Build history of the part. All positions in model axes, mm. A direction names the side the tool comes from. Give positions to 0.01 mm unless a question says otherwise; leave off trailing zeros. Write each loop counter-clockwise with the first axis right and the second up, starting at its lowest first coordinate (ties: lowest second). Pieces come first, ordered by that corner, then holes. Notation, with made-up numbers: (8.25, 70.25) - (42.25, 70.25) arc R29 cw to (42.25, 98.25) - close; hole circle Ø5 at (-30, 32.25). An arc over 180 degrees is marked (long way). Use one line per item in the form item = value. Start each with the question number.
from build123d import *

# Parameters (mm, degrees)
SKICA2_W                 = 63.5
SKICA2_H                 = 53.6
P_IDAT_VYSUNUT_M1_DEPTH  = 5
SKICA3_W                 = 63.5
SKICA3_H                 = 13
P_IDAT_VYSUNUT_M2_DEPTH  = 7.4
SKICA5_R                 = 8.5
ODEBRAT_VYSUNUT_M1_DEPTH = 74
ZKOSEN_1_SIZE            = 3
ZKOSEN_1_SIZE_2          = 3.575260778
ZAOBLIT1_R               = 2


with BuildPart() as part:
    # Skica2 → Přidat vysunutím1 (new body)
    with BuildSketch(Plane.XY):
        with Locations((6.211756064, 35.331333862)):
            Rectangle(SKICA2_W, SKICA2_H)
    extrude(amount=P_IDAT_VYSUNUT_M1_DEPTH)

    # Skica3 → Přidat vysunutím2 (add)
    with BuildSketch(Plane.XY.offset(5)):
        with Locations((6.211756064, 15.031333862)):
            Rectangle(SKICA3_W, SKICA3_H)
    extrude(amount=P_IDAT_VYSUNUT_M2_DEPTH)

    # Skica5 → Odebrat vysunutím1 (cut)
    with BuildSketch(Plane(origin=(0, 0, 0), x_dir=(-1, 0, 0), z_dir=(0, 0, -1))):
        with Locations((-17.961756064, 30.531333862)):
            Circle(SKICA5_R)
        with Locations((8.538243936, 30.531333862)):
            Circle(SKICA5_R)
    extrude(amount=-ODEBRAT_VYSUNUT_M1_DEPTH, mode=Mode.SUBTRACT)

    # Zkosení1
    # the kernel refuses this chamfer: 3.575260778, 3 mm, written as the material it takes off along each edge
    with BuildSketch(Plane(origin=(17.961756064, 30.531333862, 5), x_dir=(-1, 0, 0), z_dir=(0, -1, 0))) as zkosen_1_piece_1_section:
        Polygon((8.5 + ZKOSEN_1_SIZE, 0), (8.5, ZKOSEN_1_SIZE_2), (8.5, 0), align=None)
    zkosen_1_piece_1 = revolve(axis=Axis((17.961756064, 30.531333862, 5), (0, 0, -1)), mode=Mode.PRIVATE)
    zkosen_1_piece_1 = split(zkosen_1_piece_1, bisect_by=Plane(origin=(27.909166998, 21.531333862, 3.256497077), z_dir=(0, 1, 0)), keep=Keep.TOP, mode=Mode.PRIVATE)
    add(zkosen_1_piece_1, mode=Mode.SUBTRACT)
    with BuildSketch(Plane(origin=(-8.538243936, 30.531333862, 5), x_dir=(-1, 0, 0), z_dir=(0, -1, 0))) as zkosen_1_piece_2_section:
        Polygon((8.5 + ZKOSEN_1_SIZE, 0), (8.5, ZKOSEN_1_SIZE_2), (8.5, 0), align=None)
    zkosen_1_piece_2 = revolve(axis=Axis((-8.538243936, 30.531333862, 5), (0, 0, -1)), mode=Mode.PRIVATE)
    zkosen_1_piece_2 = split(zkosen_1_piece_2, bisect_by=Plane(origin=(1.409166998, 21.531333862, 3.256497077), z_dir=(0, 1, 0)), keep=Keep.TOP, mode=Mode.PRIVATE)
    add(zkosen_1_piece_2, mode=Mode.SUBTRACT)

    # Zaoblit1
    # the kernel refuses this fillet: 2 mm, written as the material it takes off along each edge
    with BuildSketch(Plane(origin=(17.961756064, 30.531333862, 0), x_dir=(-1, 0, 0), z_dir=(0, -1, 0))) as zaoblit1_piece_1:
        with BuildLine():
            CenterArc((10.415482978, -2), ZAOBLIT1_R, 90, 73.283856072)
            Line((8.5, -1.424739222), (8.46169034, -1.413234006))
            ThreePointArc((8.46169034, -1.413234006), (8.46, -0.712369611), (8.46, 0))
            Line((8.46, 0), (8.5, 0.04))
            Line((8.5, 0.04), (10.415482978, 0.04))
            Line((10.415482978, 0.04), (10.415482978, 0))
        make_face()
    revolve(axis=Axis((17.961756064, 30.531333862, 0), (0, 0, -1)), mode=Mode.SUBTRACT)
    with BuildSketch(Plane(origin=(-8.538243936, 30.531333862, 0), x_dir=(-1, 0, 0), z_dir=(0, -1, 0))) as zaoblit1_piece_2:
        with BuildLine():
            CenterArc((10.415482978, -2), ZAOBLIT1_R, 90, 73.283856072)
            Line((8.5, -1.424739222), (8.46169034, -1.413234006))
            ThreePointArc((8.46169034, -1.413234006), (8.46, -0.712369611), (8.46, 0))
            Line((8.46, 0), (8.5, 0.04))
            Line((8.5, 0.04), (10.415482978, 0.04))
            Line((10.415482978, 0.04), (10.415482978, 0))
        make_face()
    revolve(axis=Axis((-8.538243936, 30.531333862, 0), (0, 0, -1)), mode=Mode.SUBTRACT)


solid = part.part
(1) Cut at C-C, the plane y = 26. State how many separate pieces and enclosed holes the cut face has, then the cut area to 3 significant figures.
(2) Wall check: line 1 (X direction, y = 26, z = 2.5); line 2 (Z direction, x = 3, y = 44.5); line 3 (X direction, y = 36, z = 0.5). Give the ranges that are in metal, low to high. Write a range as from..to.
(3) Cut at A-A, the plane x = 5.5. Give the cut face in (y, z), then the cut area to 3 significant figures.
(4) Pin check, flat tips, straight feed: pin 1 Ø5 at (y, z) = (52, 9) entering from +X; pin 2 Ø4 at (x, z) = (-3.5, 8.5) entering from +Y. Stop position of each tip, or through.
(5) Cut at B-B, the plane z = 4.25. Give the cut face in (x, y), then the cut area to 3 significant figures.
(6) Cut at D-D, the plane z = 7.5. Give the cut face in (x, y), then the cut area to 4 significant figures.
(7) Which spindle directions (+Z, -Z, +X, -X, +Y, -Y) get a long thin tool onto all of the face, cutting with end or side? Do faces 1 (the flat face through (6, 47, 5)), 2 (the flat face through (6, 36, 0)), 3 (the flat face through (6, 21.531, 8)). Say none if no direction does.
(8) Two-plate mould, pull along Y, no slides. Class faces 4 (the conical face through (19.087, 39.103, 1.598)), 5 (the flat face through (6, 62.131, 2)), 6 (the flat face through (37.962, 29, 3)): +Y half, -Y half, draft (parallel to the pull), parting line (faces both ways), or undercut.
Solution:
q1.separate_pieces = 3
q1.enclosed_holes = 0
q1.area = 146 mm2
q2.line_1 = -25.54..-16.78, -0.3..9.72, 26.2..37.96
q2.line_2 = 0..5
q2.line_3 = -25.54..-15.8, -1.27..10.7, 25.23..37.96
q3.outline = (8.53, 0) - (62.13, 0) - (62.13, 5) - (21.53, 5) - (21.53, 12.4) - (8.53, 12.4) - close
q3.area = 364 mm2
q4.pin_1 = through
q4.pin_2 = 21.53
q5.outline = (-25.54, 8.53) - (37.96, 8.53) - (37.96, 62.13) - (-25.54, 62.13) - close; hole (-14.64, 21.53) - (-2.44, 21.53) arc R10.87 ccw (long way) to start; hole (11.86, 21.53) - (24.06, 21.53) arc R10.87 ccw (long way) to start
q5.area = 2,690 mm2
q6.outline = (-25.54, 8.53) - (37.96, 8.53) - (37.96, 21.53) - (-25.54, 21.53) - close
q6.area = 825.5 mm2
q7.face_1 = +Z, +X, -X, +Y
q7.face_2 = -Z, +X, -X, +Y, -Y
q7.face_3 = +Z
q8.face_4 = undercut
q8.face_5 = +Y half
q8.face_6 = draft
